from build123d import *

# Parameters (mm, degrees)
SKETCH_1_R      = 1.25
EXTRUDE_1_DEPTH = 8
FILLET_1_R      = 0.5


with BuildPart() as part:
    # 草图1 → 凸台-拉伸1 (new body)
    with BuildSketch(Plane(origin=(0, 0, 0), x_dir=(1, 0, 0), z_dir=(0, 1, 0))):
        with BuildLine():
            Line((-22.9, 33.888050991), (-22.9, 2.142428529))
            ThreePointArc((-22.9, 2.142428529), (-21.006975687, 9.365200078), (-16.9, 15.600961509))
            Line((-16.9, 15.600961509), (-16.9, 37.24513391))
            ThreePointArc((-16.9, 37.24513391), (-19.970666024, 35.692891429), (-22.9, 33.888050991))
        make_face()
        with Locations((-19.9, 28.931907268)):
            Circle(SKETCH_1_R, mode=Mode.SUBTRACT)
        with Locations((-19.9, 18.931907268)):
            Circle(SKETCH_1_R, mode=Mode.SUBTRACT)
    extrude(amount=EXTRUDE_1_DEPTH)

    # 圆角1
    fillet_1_edges = [part.edges().sort_by_distance(p)[0] for p in [
        (-22.9, 4, -2.142428529),
    ]]
    fillet(fillet_1_edges, radius=FILLET_1_R)


solid = part.part
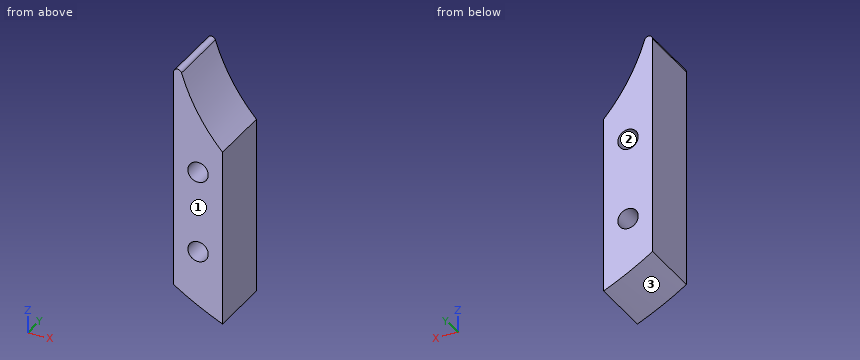
Model file for the job. Use its own axes, mm. Face numbers are marked on the shaded views. Give positions to 0.01 mm unless a question says otherwise; leave off trailing zeros. Loops run counter-clockwise (first coordinate to the right, second up) from the corner with the lowest first, then second, coordinate; pieces in that order, holes last.
1) Saw through at B-B (y = 4.5). Write the cut outline in (x, z), plus the area to 3 significant figures.
2) Flat gauge pin, fed straight in: pin 1 Ø3 at (x, y) = (-20, 7) entering from -Z. Where does the tip first touch, or does it go through?
3) Saw through at D-D (x = -21.5). Write the cut outline in (y, z).
4) Wall check: line 1 (Z direction, x = -19.9, y = 4.75); line 2 (Z direction, x = -20.5, y = 1); line 3 (X direction, y = 1, z = -19). Give the ranges that are in metal, low to high.
5) Pull direction X, two halves, no side cores. Call the marked faces 1, 2 and 3: +X half, -X half, draft (parallel to the pull), parting line (faces both ways), or undercut.
6) Saw through at C-C (z = -10). Write the cut outline in (x, y).
7) Saw through at A-A (x = -19.9). Write the cut outline in (y, z).
Answer block:
1. outline: (-22.9, -33.89) arc R40.9 ccw to (-16.9, -37.25) - (-16.9, -15.6) arc R23 cw to (-21.92, -6.95) arc R0.5 ccw to (-22.9, -7.11) - close; hole circle Ø2.5 at (-19.9, -28.93); hole circle Ø2.5 at (-19.9, -18.93)
1. area: 137 mm2
2. pin 1: stops at z = -36.48
3. outline: (0, -34.79) - (8, -34.79) - (8, -8.17) - (0, -8.17) - close
4. line 1: z = -35.73 to -30.18, -27.68 to -20.18, -17.68 to -11.53
4. line 2: z = -35.39 to -30.03, -27.84 to -20.03, -17.84 to -10.43
4. line 3: x = -22.9 to -21.15, -18.65 to -16.9
5. face 1: draft
5. face 2: undercut
5. face 3: -X half
6. outline: (-22.9, 0) - (-20.71, 0) - (-20.71, 8) - (-22.9, 8) - close
7. outline: (0, -35.73) - (8, -35.73) - (8, -30.18) - (0, -30.18) - close; (0, -27.68) - (8, -27.68) - (8, -20.18) - (0, -20.18) - close; (0, -17.68) - (8, -17.68) - (8, -11.53) - (0, -11.53) - close
